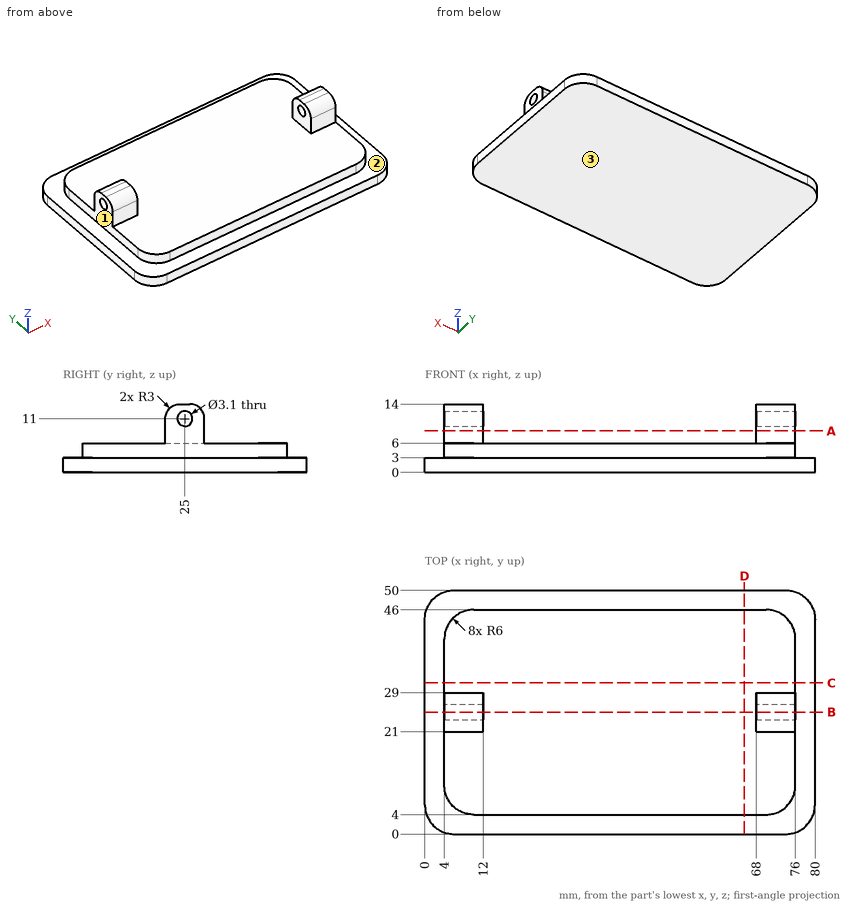
Job drawing, mm, ordinate dimensions from the low corner. One solid piece. A direction names the side the tool comes from. Round coordinates to 2 decimals unless told otherwise and drop trailing zeros. Loops run counter-clockwise (first coordinate to the right, second up) from the corner with the lowest first, then second, coordinate; pieces in that order, holes last.
Item 1: Cut at A-A, the plane z = 8.5. Give the cut face in (x, y).
Item 2: Cut at D-D, the plane x = 65.5. Give the cut face in (y, z).
Item 3: Drill centre lines: line 1 (Z direction, x = 5, y = 25); line 2 (X direction, y = 27.5, z = 10.5); line 3 (Y direction, x = 32.5, z = 3.25). Where is each one in solid material? Low to high.
Item 4: Cut at B-B, the plane y = 25. Give the cut face in (x, z), then the cut area to 3 significant figures.
Item 5: 3-axis set-ups, long thin cutter, end or side, ignore diameter. For the marked faces 1, 2 and 3: which of +Z, -Z, +X, -X, +Y, -Y reach the whole face in a straight line?
Item 6: Cut at C-C, the plane y = 31. Give the cut face in (x, z), then the cut area to 3 significant figures.
Item 7: Drop flat-ended pins along their axis: P1, Ø2.5, axis at x = 8, z = 8.5, coming from the +Y side; P2, Ø4, axis at x = 32.5, y = 33, coming from the +Z side; P3, Ø2.5, axis at x = 9.5, z = 7.5, coming from the -Y side. Give the stop position or say it passes through.
A:
1. outline: (4, 21) - (12, 21) - (12, 29) - (4, 29) - close; (68, 21) - (76, 21) - (76, 29) - (68, 29) - close
2. outline: (0, 0) - (50, 0) - (50, 3) - (46, 3) - (46, 6) - (4, 6) - (4, 3) - (0, 3) - close
3. line 1: z = 0 to 9.45, 12.55 to 14
3. line 2: x = 4 to 12, 68 to 76
3. line 3: y = 4 to 46
4. outline: (0, 0) - (80, 0) - (80, 3) - (76, 3) - (76, 9.45) - (68, 9.45) - (68, 6) - (12, 6) - (12, 9.45) - (4, 9.45) - (4, 3) - (0, 3) - close; (4, 12.55) - (12, 12.55) - (12, 14) - (4, 14) - close; (68, 12.55) - (76, 12.55) - (76, 14) - (68, 14) - close
4. area: 534 mm2
5. face 1: +Z, -X, +Y, -Y
5. face 2: +Z
5. face 3: -Z, +X, -X, +Y, -Y
6. outline: (0, 0) - (80, 0) - (80, 3) - (76, 3) - (76, 6) - (4, 6) - (4, 3) - (0, 3) - close
6. area: 456 mm2
7. P1: stops at y = 29
7. P2: stops at z = 6
7. P3: stops at y = 21
